CAD build for the part. Positions are in the model's coordinates, mm. A direction names the side the tool comes from. Give positions to 0.01 mm unless a question says otherwise; leave off trailing zeros. Loops run counter-clockwise (first coordinate to the right, second up) from the corner with the lowest first, then second, coordinate; pieces in that order, holes last. Notation, with made-up numbers: (50, -18) - (57, -18) arc R25 cw to (57, 10) - close; hole circle Ø9 at (63.25, 43.5). An arc over 180 degrees is marked (long way). Return JSON: item names as keys, results as strings.
from build123d import *

# Parameters (mm, degrees)
EXTRUDE_1_DEPTH       = 172
SHELL_START           = 6
SHELL_1_DEPTH         = 160
SKETCH_2_W            = 36
SKETCH_2_H            = 16
CUT_EXTRUDE_1_DEPTH   = 74
EXTRUDE_2_DEPTH       = 2
SKETCH_4_R            = 10
CUT_EXTRUDE_2_DEPTH   = 186
SKETCH_5_R            = 1.5
CUT_EXTRUDE_3_DEPTH   = 10
EXTRUDE_3_DEPTH       = 172
SKETCH_7_W            = 36
SKETCH_7_H            = 16
CUT_EXTRUDE_4_DEPTH   = 172
SKETCH_8_W            = 6
SKETCH_8_H            = 172
CUT_EXTRUDE_5_DEPTH   = 3
EXTRUDE_4_DEPTH       = 15
CHAMFER_1_SIZE        = 15
CHAMFER_2_SIZE        = 15
CHAMFER_3_SIZE        = 8
SKETCH_10_R           = 1.35
CUT_EXTRUDE_6_DEPTH   = 15
SKETCH_12_R           = 1.35
CUT_EXTRUDE_7_DEPTH   = 15
SKETCH_14_OUTSIDE_W   = 213.548
SKETCH_14_OUTSIDE_H   = 97.548
SKETCH_14_OUTSIDE_W_2 = 15
SKETCH_14_OUTSIDE_H_2 = 56
CUT_EXTRUDE_8_DEPTH   = 82.5
EXTRUDE_5_DEPTH       = 15
CUT_EXTRUDE_9_DEPTH   = 15
SKETCH_17_W           = 13
SKETCH_17_H           = 5
EXTRUDE_6_DEPTH       = 15
EXTRUDE_7_DEPTH       = 20
SHELL_START_2         = 78.159554327
SHELL_2_DEPTH         = 10
EXTRUDE_8_DEPTH       = 28
CUT_EXTRUDE_10_DEPTH  = 20
CUT_EXTRUDE_11_DEPTH  = 20
CUT_EXTRUDE_12_DEPTH  = 63


# Read off the part's stored shape, not the designer's step: 抽壳1, 抽壳2
with BuildPart() as part:
    # 草图1 → 凸台-拉伸1 (new body)
    with BuildSketch(Plane.XY):
        with BuildLine():
            Line((0, 0), (0, 40))
            Line((0, 40), (-5, 40))
            Line((-5, 40), (-5, 53))
            Line((-5, 53), (-23, 53))
            Line((-23, 53), (-64.888578151, 47.050698608))
            Line((-64.888578151, 47.050698608), (-15.121320344, -2.121320344))
            ThreePointArc((-15.121320344, -2.121320344), (-14.148050297, -2.771638598), (-13, -3))
            Line((-13, -3), (-5, -3))
            Line((-5, -3), (-5, 0))
            Line((-5, 0), (0, 0))
        make_face()
    extrude(amount=EXTRUDE_1_DEPTH)

    # 抽壳1 outline → 抽壳1 (cut)
    with BuildSketch(Plane.XY.offset(SHELL_START)):
        Polygon((-11, 6), (-6, 6), (-6, 34), (-11, 34), (-11, 47), (-22.576046832, 47), (-52.061983815, 42.812206246), (-11.767841448, 3), (-11, 3), align=None)
    extrude(amount=SHELL_1_DEPTH, mode=Mode.SUBTRACT)

    # 草图2 → 切除-拉伸1 (cut)
    with BuildSketch(Plane(origin=(0, 0, 0), x_dir=(0, 0, -1), z_dir=(1, 0, 0))):
        with Locations((-136, 10)):
            Rectangle(SKETCH_2_W, SKETCH_2_H)
        with Locations((-36, 10)):
            Rectangle(SKETCH_2_W, SKETCH_2_H)
    extrude(amount=-CUT_EXTRUDE_1_DEPTH, mode=Mode.SUBTRACT)

    # 草图3 → 凸台-拉伸2 (add, symmetric)
    with BuildSketch(Plane(origin=(0, 0, 86), x_dir=(-1, 0, 0), z_dir=(0, 0, -1))):
        Polygon((5, 53), (5, 40), (0, 40), (0, 0), (5, 0), (5, -3), (13, -3), (16.579355858, -0.680723591), (64.888578151, 47.050698608), (23, 53), align=None)
    extrude(amount=EXTRUDE_2_DEPTH, both=True)

    # 草图4 → 切除-拉伸2 (cut)
    with BuildSketch(Plane.XY.offset(172)):
        with Locations((-15, 21.071297481)):
            Circle(SKETCH_4_R)
    extrude(amount=-CUT_EXTRUDE_2_DEPTH, mode=Mode.SUBTRACT)

    # 草图5 → 切除-拉伸3 (cut)
    with BuildSketch(Plane(origin=(0, 53, 0), x_dir=(1, 0, 0), z_dir=(0, 1, 0))):
        with Locations(Location((-13.338195438, -63.5, 0), (0, 0, 270))):
            Circle(SKETCH_5_R)
        with Locations(Location((-13.338195438, -108.5, 0), (0, 0, 270))):
            Circle(SKETCH_5_R)
    extrude(amount=-CUT_EXTRUDE_3_DEPTH, mode=Mode.SUBTRACT)

    # 草图6 → 凸台-拉伸3 (add)
    with BuildSketch(Plane.XY.offset(172)):
        Polygon((-11, 6), (-14.804157153, 6), (-11.767841448, 3), (-11, 3), align=None)
    extrude(amount=-EXTRUDE_3_DEPTH)

    # 草图7 → 切除-拉伸4 (cut)
    with BuildSketch(Plane(origin=(0, 0, 0), x_dir=(0, 0, -1), z_dir=(1, 0, 0))):
        with Locations((-136, 10)):
            Rectangle(SKETCH_7_W, SKETCH_7_H)
        with Locations((-36, 10)):
            Rectangle(SKETCH_7_W, SKETCH_7_H)
    extrude(amount=-CUT_EXTRUDE_4_DEPTH, mode=Mode.SUBTRACT)

    # 草图8 → 切除-拉伸5 (cut)
    with BuildSketch(Plane.XZ.offset(3)):
        with Locations((-8, 86)):
            Rectangle(SKETCH_8_W, SKETCH_8_H)
    extrude(amount=-CUT_EXTRUDE_5_DEPTH, mode=Mode.SUBTRACT)

    # 草图9 → 凸台-拉伸4 (add)
    with BuildSketch(Plane(origin=(0, 0, 0), x_dir=(0, 0, -1), z_dir=(1, 0, 0))):
        Polygon((-86, 40), (-151, 40), (-151, 35), (-86, 35), (-21, 35), (-21, 40), align=None)
    extrude(amount=EXTRUDE_4_DEPTH)

    # 倒角1
    chamfer_1_edges = [part.edges().sort_by_distance(p)[0] for p in [
        (15, 37.5, 151),
    ]]
    chamfer(chamfer_1_edges, length=CHAMFER_1_SIZE - 0.0001)  # a hair under: the kernel refuses the full size

    # 倒角2
    chamfer_2_edges = [part.edges().sort_by_distance(p)[0] for p in [
        (15, 37.5, 21),
    ]]
    chamfer(chamfer_2_edges, length=CHAMFER_2_SIZE - 0.0001)  # a hair under: the kernel refuses the full size

    # 倒角3
    chamfer_3_edges = [part.edges().sort_by_distance(p)[0] for p in [
        (0, 35, 86),
    ]]
    chamfer(chamfer_3_edges, length=CHAMFER_3_SIZE)

    # 草图10 → 切除-拉伸6 (cut)
    with BuildSketch(Plane.XZ):
        with Locations((-5, 158)):
            Circle(SKETCH_10_R)
        with Locations((-5, 111)):
            Circle(SKETCH_10_R)
        with Locations((-5, 61)):
            Circle(SKETCH_10_R)
        with Locations((-5, 14.01360213)):
            Circle(SKETCH_10_R)
    extrude(amount=-CUT_EXTRUDE_6_DEPTH, mode=Mode.SUBTRACT)

    # 草图12 → 切除-拉伸7 (cut)
    with BuildSketch(Plane(origin=(0, 40, 0), x_dir=(1, 0, 0), z_dir=(0, 1, 0))):
        with Locations(Location((5, -41, 0), (0, 0, 270))):
            Circle(SKETCH_12_R)
        with Locations(Location((5, -86, 0), (0, 0, 270))):
            Circle(SKETCH_12_R)
        with Locations(Location((5, -131, 0), (0, 0, 270))):
            Circle(SKETCH_12_R)
    extrude(amount=-CUT_EXTRUDE_7_DEPTH, mode=Mode.SUBTRACT)

    # 草图14 outside → 切除-拉伸8 (cut, symmetric)
    with BuildSketch(Plane(origin=(0, 0, 0), x_dir=(0, 0, -1), z_dir=(1, 0, 0))):
        with Locations((-86, 25)):
            Rectangle(SKETCH_14_OUTSIDE_W, SKETCH_14_OUTSIDE_H)
        with Locations((-75.659554327, 25)):
            Rectangle(SKETCH_14_OUTSIDE_W_2, SKETCH_14_OUTSIDE_H_2, mode=Mode.SUBTRACT)
    extrude(amount=CUT_EXTRUDE_8_DEPTH, both=True, mode=Mode.SUBTRACT)

    # 草图15 → 凸台-拉伸5 (add)
    with BuildSketch(Plane(origin=(0, 0, 68.159554327), x_dir=(-1, 0, 0), z_dir=(0, 0, -1))):
        Polygon((0, 0), (-2, 0), (-2, 29), (0, 27), align=None)
    extrude(amount=-EXTRUDE_5_DEPTH)

    # 草图16 → 切除-拉伸9 (cut)
    with BuildSketch(Plane(origin=(0, 0, 68.159554327), x_dir=(-1, 0, 0), z_dir=(0, 0, -1))):
        Polygon((-2, 29), (-2, 35), (-8, 35), align=None)
    extrude(amount=-CUT_EXTRUDE_9_DEPTH, mode=Mode.SUBTRACT)

    # 草图17 → 凸台-拉伸6 (add)
    with BuildSketch(Plane(origin=(0, 0, 68.159554327), x_dir=(-1, 0, 0), z_dir=(0, 0, -1))):
        with Locations((-8.5, 32.5)):
            Rectangle(SKETCH_17_W, SKETCH_17_H)
    extrude(amount=-EXTRUDE_6_DEPTH)

    # 草图18 → 凸台-拉伸7 (add)
    with BuildSketch(Plane(origin=(0, 0, 68.159554327), x_dir=(-1, 0, 0), z_dir=(0, 0, -1))):
        with BuildLine():
            Line((-15, 40), (-15, 30))
            Line((-15, 30), (-2, 30))
            Line((-2, 30), (-2, 0))
            Line((-2, 0), (11, 0))
            Line((11, 0), (11, -3))
            Line((11, -3), (13, -3))
            ThreePointArc((13, -3), (14.148050297, -2.771638598), (15.121320344, -2.121320344))
            Line((15.121320344, -2.121320344), (64.888578151, 47.050698608))
            Line((64.888578151, 47.050698608), (23, 53))
            Line((23, 53), (5, 53))
            Line((5, 53), (5, 40))
            Line((5, 40), (-15, 40))
        make_face()
    extrude(amount=-EXTRUDE_7_DEPTH)

    # 抽壳2 outline → 抽壳2 (cut)
    with BuildSketch(Plane.XY.offset(SHELL_START_2)):
        Polygon((-8, 30), (-15, 30), (-15, 43), (-22.293411387, 43), (-43.510920925, 39.986544671), (-13.161382076, 10), (-8, 10), align=None)
    extrude(amount=SHELL_2_DEPTH, mode=Mode.SUBTRACT)

    # 草图20 → 凸台-拉伸8 (add)
    with BuildSketch(Plane.XY.offset(88.159554327)):
        Polygon((15, 40), (-15, 40), (-15, 30), (-8, 30), (-8, 22), (2, 22), (2, 30), (15, 30), align=None)
    extrude(amount=EXTRUDE_8_DEPTH)

    # 草图21 → 切除-拉伸10 (cut)
    with BuildSketch(Plane(origin=(2, 0, 0), x_dir=(0, 0, -1), z_dir=(1, 0, 0))):
        Polygon((-116.159554327, 30), (-88.159554327, 22), (-116.159554327, 22), align=None)
    extrude(amount=-CUT_EXTRUDE_10_DEPTH, mode=Mode.SUBTRACT)

    # 草图22 → 切除-拉伸11 (cut)
    with BuildSketch(Plane(origin=(0, 40, 0), x_dir=(1, 0, 0), z_dir=(0, 1, 0))):
        Polygon((-8, -116.159554327), (-15, -116.159554327), (-15, -88.159554327), (-5, -116.159554327), align=None)
    extrude(amount=-CUT_EXTRUDE_11_DEPTH, mode=Mode.SUBTRACT)


with BuildPart() as body_2:
    # 镜向6: mirrored copy
    add(part.part.mirror(Plane.XY.offset(126.159554327)))


with BuildPart() as part_1:
    add(part.part)

    # 草图24 → 切除-拉伸12 (cut, symmetric)
    with BuildSketch(Plane(origin=(0, 40, 0), x_dir=(1, 0, 0), z_dir=(0, 1, 0))):
        Polygon((-102.39415219, -125.726561749), (32.776263332, -125.726561749), (42.64807393, -30.561512846), (-60.072475676, -35.644094183), align=None)
    extrude(amount=CUT_EXTRUDE_12_DEPTH, both=True, mode=Mode.SUBTRACT)


solid = body_2.part
1. Pull direction X, two halves, no side cores. Call faces 5 (the face through (-40.353, 22.809, 174.3)), 6 (the face through (-5, 0, 174)), 7 (the face through (-11, 10, 169)): +X half, -X half, draft (parallel to the pull), parting line (faces both ways), or undercut.
Values follow:
{"face 5": "-X half", "face 6": "draft", "face 7": "undercut"}
2. Cut at A-A, the plane z = 169.5. Write the cut outline in (x, y), plus the area to 3 significant figures.
Values follow:
{"outline": "(-64.89, 47.05) - (-15.12, -2.12) arc R3 ccw to (-13, -3) - (-11, -3) - (-11, 0) - (2, 0) - (2, 30) - (15, 30) - (15, 40) - (-5, 40) - (-5, 53) - (-23, 53) - close; hole (-43.51, 39.99) - (-13.16, 10) - (-8, 10) - (-8, 30) - (-15, 30) - (-15, 43) - (-22.29, 43) - close", "area": "1,760 mm²"}
3. Drill centre lines: probe 1 along Y at (x, z) = (-6.5, 179); probe 2 along Z at (x, y) = (-40, 37.5); probe 3 along Y at (x, z) = (0, 181.5). Where is each one in solid material? Low to high.
Values follow:
{"probe 1": "y = 0 to 53", "probe 2": "z = 174.16 to 184.16", "probe 3": "y = 0 to 40"}
4. Cut at B-B, the plane y = 18. Write the cut outline in (x, z).
Values follow:
{"outline": "(-35.49, 164.16) - (-21.26, 164.16) - (-21.26, 174.16) - (-8, 174.16) - (-8, 164.16) - (2, 164.16) - (2, 184.16) - (-35.49, 184.16) - close"}
5. Cut at C-C, the plane z = 177. Write the cut outline in (x, y), plus the area to 3 significant figures.
Values follow:
{"outline": "(-64.89, 47.05) - (-15.12, -2.12) arc R3 ccw to (-13, -3) - (-11, -3) - (-11, 0) - (2, 0) - (2, 30) - (15, 30) - (15, 40) - (-5, 40) - (-5, 53) - (-23, 53) - close", "area": "2,350 mm²"}
6. Which spindle directions (+Z, -Z, +X, -X, +Y, -Y) get a long thin tool onto all of the face, cutting with end or side? Do faces 1 (the face through (-43.651, 50.067, 174.3)), 2 (the face through (2, 18, 171)), 3 (the face through (-5, 47, 174)), 4 (the face through (-28.549, 25.203, 169.23)). Say none if no direction does.
Values follow:
{"face 1": "+Z, -Z, -X, +Y", "face 2": "+Z, -Z, +X, -Y", "face 3": "+Z, -Z, +X, +Y", "face 4": "-Z"}
7. Cut at D-D, the plane x = -38. Write the cut outline in (y, z), plus the area to 3 significant figures.
Values follow:
{"outline": "(20.48, 164.16) - (34.54, 164.16) - (34.54, 174.16) - (40.77, 174.16) - (40.77, 164.16) - (50.87, 164.16) - (50.87, 184.16) - (20.48, 184.16) - close", "area": "545 mm²"}
8. Drop flat-ended pins along their axis: P1, Ø10.5, axis at x = -5, z = 178, coming from the -Y side; P2, Ø4, axis at x = -46, z = 171, coming from the +Y side; P3, Ø2.5, axis at y = -2, z = 176.5, coming from the +X side; P4, Ø15, axis at x = -3.5, z = 169, coming from the +Y side. Give the stop position or say it passes through.
Values follow:
{"P1": "stops at y = 0", "P2": "stops at y = 50.02", "P3": "stops at x = -11", "P4": "stops at y = 53"}
